Check sheet for the modelled part. Datum: model origin and axes. Units: mm. Round coordinates to 2 decimals unless told otherwise and drop trailing zeros. Loops run counter-clockwise (first coordinate to the right, second up) from the corner with the lowest first, then second, coordinate; pieces in that order, holes last. Notation, with made-up numbers: (61, 78) -> (72, 78) arc R18 ccw to (72, 94) -> close; hole circle Ø11 at (-18.75, 12.25). An arc over 180 degrees is marked (long way). One line per item, written item: value. Start each with the question number.
1. Cross-section at C-C on z = 58.25. Count the separate pieces of the cut face and the enclosed holes in it, then the cut area to 3 significant figures.
2. Release check for a two-part mould opening along Y. For faces 1 (the face through (-39.169, 127.403, 58.479)), 2 (the face through (-1, 114, 57)) record: +Y half, -Y half, draft (parallel to the pull), parting line (faces both ways), or undercut.
3. Material ranges on L1, parallel to X at y = 149.5, z = 57.55; L2, parallel to X at y = 70, z = 57.7; L3, parallel to Y at x = -15, z = 59.15, recorded low to high.
4. Cross-section at B-B on x = -30. Record the cut outline in (y, z), then the cut area to 3 significant figures.
5. Cross-section at A-A on y = 40. Record the cut outline in (x, z), then the cut area to 3 significant figures.
from build123d import *

# Parameters (mm, degrees)
CYLINDER004_R     = 1.8
CYLINDER004_DEPTH = 200
ARRAY003_X_COUNT  = 9
ARRAY003_X_PITCH  = 10
ARRAY003_Y_COUNT  = 2
ARRAY003_Y_PITCH  = 146
BOX011_W          = 50
BOX011_H          = 50
BOX011_DEPTH      = 100
CYLINDER012_R     = 1.8
CYLINDER012_DEPTH = 100
ARRAY008_X_COUNT  = 5
ARRAY008_X_PITCH  = 10
ARRAY008_Y_COUNT  = 13
ARRAY008_Y_PITCH  = 10
CYLINDER011_R     = 18.5
CYLINDER011_DEPTH = 100
CYLINDER010_R     = 1.9
CYLINDER010_DEPTH = 100
ARRAY007_X_COUNT  = 2
ARRAY007_X_PITCH  = 32
ARRAY007_Y_COUNT  = 2
ARRAY007_Y_PITCH  = 32
CYLINDER006_R     = 1.8
CYLINDER006_DEPTH = 200
ARRAY005_X_COUNT  = 2
ARRAY005_X_PITCH  = 80
ARRAY005_Y_COUNT  = 10
ARRAY005_Y_PITCH  = 10
BOX009_W          = 96
BOX009_H          = 180
BOX009_DEPTH      = 3


with BuildPart() as psu_bottom_bolt_hole_array:
    # Cylinder004 → Cylinder004 (new body)
    with BuildSketch(Plane(origin=(-40, 20, 0), x_dir=(1, 0, 0), z_dir=(0, 0, 1))):
        Circle(CYLINDER004_R)
    extrude(amount=CYLINDER004_DEPTH)

    # Array003 X: psu bottom bolt hole array ×9


with BuildPart() as psu_bottom_bolt_hole_array_1:
    add(psu_bottom_bolt_hole_array.part)
    with Locations(*[(i * ARRAY003_X_PITCH, 0, 0) for i in range(1, ARRAY003_X_COUNT)]):
        add(psu_bottom_bolt_hole_array.part)

    # Array003 Y: psu bottom bolt hole array ×2


with BuildPart() as psu_bottom_bolt_hole_array_2:
    add(psu_bottom_bolt_hole_array_1.part)
    with Locations(*[(0, i * ARRAY003_Y_PITCH, 0) for i in range(1, ARRAY003_Y_COUNT)]):
        add(psu_bottom_bolt_hole_array_1.part)


with BuildPart() as no_vent_hole_cube:
    # Box011 → Box011 (new body)
    with BuildSketch(Plane(origin=(-25, 66, 0), x_dir=(1, 0, 0), z_dir=(0, 0, 1))):
        with Locations((25, 25)):
            Rectangle(BOX011_W, BOX011_H)
    extrude(amount=BOX011_DEPTH)


with BuildPart() as vent_holes_cut:
    # Cylinder012 → Cylinder012 (new body)
    with BuildSketch(Plane.XY):
        Circle(CYLINDER012_R)
    extrude(amount=CYLINDER012_DEPTH)

    # Array008 X: vent holes cut ×5


with BuildPart() as vent_holes_cut_1:
    add(vent_holes_cut.part)
    with Locations(*[(i * ARRAY008_X_PITCH, 0, 0) for i in range(1, ARRAY008_X_COUNT)]):
        add(vent_holes_cut.part)

    # Array008 Y: vent holes cut ×13


with BuildPart() as vent_holes_cut_2:
    add(vent_holes_cut_1.part)
    with Locations(*[(0, i * ARRAY008_Y_PITCH, 0) for i in range(1, ARRAY008_Y_COUNT)]):
        add(vent_holes_cut_1.part)


with BuildPart() as vent_holes_cut_3:
    # Array008 placement: moved
    add(vent_holes_cut_2.part.moved(Location((-20, 30, 0))))

    # Cut012: cut no vent hole cube
    add(no_vent_hole_cube.part, mode=Mode.SUBTRACT)


with BuildPart() as fan_hole:
    # Cylinder011 → Cylinder011 (new body)
    with BuildSketch(Plane.XY):
        Circle(CYLINDER011_R)
    extrude(amount=CYLINDER011_DEPTH)


with BuildPart() as fan_hole_fusion:
    # Cylinder010 → Cylinder010 (new body)
    with BuildSketch(Plane.XY):
        Circle(CYLINDER010_R)
    extrude(amount=CYLINDER010_DEPTH)

    # Array007 X: fan hole fusion ×2


with BuildPart() as fan_hole_fusion_1:
    add(fan_hole_fusion.part)
    with Locations(*[(i * ARRAY007_X_PITCH, 0, 0) for i in range(1, ARRAY007_X_COUNT)]):
        add(fan_hole_fusion.part)

    # Array007 Y: fan hole fusion ×2


with BuildPart() as fan_hole_fusion_2:
    add(fan_hole_fusion_1.part)
    with Locations(*[(0, i * ARRAY007_Y_PITCH, 0) for i in range(1, ARRAY007_Y_COUNT)]):
        add(fan_hole_fusion_1.part)


with BuildPart() as fan_hole_fusion_3:
    # Array007 placement: moved
    add(fan_hole_fusion_2.part.moved(Location((-16, -16, 0))))

    # Fusion011: union fan hole
    add(fan_hole.part)


with BuildPart() as fan_hole_fusion_4:
    # Fusion011 placement: moved
    add(fan_hole_fusion_3.part.moved(Location((0, 90, 0))))


with BuildPart() as top_hole_fusion:
    # Cylinder006 → Cylinder006 (new body)
    with BuildSketch(Plane(origin=(-40, 9, 0), x_dir=(1, 0, 0), z_dir=(0, 0, 1))):
        Circle(CYLINDER006_R)
    extrude(amount=CYLINDER006_DEPTH)

    # Array005 X: top hole fusion ×2


with BuildPart() as top_hole_fusion_1:
    add(top_hole_fusion.part)
    with Locations(*[(i * ARRAY005_X_PITCH, 0, 0) for i in range(1, ARRAY005_X_COUNT)]):
        add(top_hole_fusion.part)

    # Array005 Y: top hole fusion ×10


with BuildPart() as top_hole_fusion_2:
    add(top_hole_fusion_1.part)
    with Locations(*[(0, i * ARRAY005_Y_PITCH, 0) for i in range(1, ARRAY005_Y_COUNT)]):
        add(top_hole_fusion_1.part)


with BuildPart() as top_hole_fusion_3:
    # Array005 placement: moved
    add(top_hole_fusion_2.part.moved(Location((0, 40, 0))))

    # Fusion012: union psu bottom bolt hole array, vent holes cut, fan hole fusion
    add(psu_bottom_bolt_hole_array_2.part)
    add(vent_holes_cut_3.part)
    add(fan_hole_fusion_4.part)


with BuildPart() as psu_top_cut:
    # Box009 → Box009 (new body)
    with BuildSketch(Plane(origin=(-48, 3, 57), x_dir=(1, 0, 0), z_dir=(0, 0, 1))):
        with Locations((48, 90)):
            Rectangle(BOX009_W, BOX009_H)
    extrude(amount=BOX009_DEPTH)

    # Cut010: cut top hole fusion
    add(top_hole_fusion_3.part, mode=Mode.SUBTRACT)


solid = psu_top_cut.part
Taken from the geometry:
1. separate pieces: 1
1. enclosed holes: 83
1. area: 15,400 mm2
2. face 1: undercut
2. face 2: draft
3. L1: x = -48 to -21.73, -18.27 to -11.73, -8.27 to -1.73, 1.73 to 8.27, 11.73 to 18.27, 21.73 to 48
3. L2: x = -48 to -41.5, -38.5 to 38.5, 41.5 to 48
3. L3: y = 3 to 72.38, 75.62 to 79.17, 100.83 to 104.38, 107.62 to 183
4. outline: (3, 57) -> (18.2, 57) -> (18.2, 60) -> (3, 60) -> close; (21.8, 57) -> (164.2, 57) -> (164.2, 60) -> (21.8, 60) -> close; (167.8, 57) -> (183, 57) -> (183, 60) -> (167.8, 60) -> close
4. area: 518 mm2
5. outline: (-48, 57) -> (-21.8, 57) -> (-21.8, 60) -> (-48, 60) -> close; (-18.2, 57) -> (-11.8, 57) -> (-11.8, 60) -> (-18.2, 60) -> close; (-8.2, 57) -> (-1.8, 57) -> (-1.8, 60) -> (-8.2, 60) -> close; (1.8, 57) -> (8.2, 57) -> (8.2, 60) -> (1.8, 60) -> close; (11.8, 57) -> (18.2, 57) -> (18.2, 60) -> (11.8, 60) -> close; (21.8, 57) -> (48, 57) -> (48, 60) -> (21.8, 60) -> close
5. area: 234 mm2
